```python
from build123d import *

# Parameters (mm, degrees)
RESSALTO_EXTRUS_O1_DEPTH = 17
ESBO_O2_W                = 18
ESBO_O2_H                = 13
CORTE_EXTRUS_O1_DEPTH    = 18
ESBO_O3_R                = 3
CORTE_EXTRUS_O2_DEPTH    = 2
ESBO_O4_R                = 3
CORTE_EXTRUS_O3_DEPTH    = 3


with BuildPart() as part:
    # Esboço1 → Ressalto-extrusão1 (new body)
    with BuildSketch(Plane.XY):
        Polygon((0, 0), (0, 20), (2, 20), (20, 2), (20, 0), align=None)
    extrude(amount=RESSALTO_EXTRUS_O1_DEPTH)

    # Esboço2 → Corte-extrusão1 (cut)
    with BuildSketch(Plane(origin=(0, 20, 0), x_dir=(1, 0, 0), z_dir=(0, 1, 0))):
        with Locations((11, -8.5)):
            Rectangle(ESBO_O2_W, ESBO_O2_H)
    extrude(amount=-CORTE_EXTRUS_O1_DEPTH, mode=Mode.SUBTRACT)

    # Esboço3 → Corte-extrusão2 (cut)
    with BuildSketch(Plane(origin=(2, 0, 0), x_dir=(0, 0, -1), z_dir=(1, 0, 0))):
        with Locations((-8.5, 11)):
            Circle(ESBO_O3_R)
    extrude(amount=-CORTE_EXTRUS_O2_DEPTH, mode=Mode.SUBTRACT)

    # Esboço4 → Corte-extrusão3 (cut, through all)
    with BuildSketch(Plane(origin=(0, 2, 0), x_dir=(1, 0, 0), z_dir=(0, 1, 0))):
        with Locations((11, -8.5)):
            Circle(ESBO_O4_R)
    extrude(amount=-CORTE_EXTRUS_O3_DEPTH, mode=Mode.SUBTRACT)


solid = part.part
```
Work out the finished part from the listing and answer in its coordinate system (mm). A direction names the side the tool comes from. Give positions to 0.01 mm unless a question says otherwise; leave off trailing zeros. Loops run counter-clockwise (first coordinate to the right, second up) from the corner with the lowest first, then second, coordinate; pieces in that order, holes last. Notation, with made-up numbers: (-13.75, 60) - (35.25, 60) arc R14 ccw to (35.25, 72) - close; hole circle Ø6 at (7.25, -24.75). An arc over 180 degrees is marked (long way). Use CSV: the item, a comma, the result in double quotes. Start each with the question number.
(1) Find section C-C, the plane y = 4. Determine the outline of the cut face in (x, z).
(2) Find the intervals of material crossed by L1, parallel to Z at x = 11.5, y = 6.5; L2, parallel to Z at x = 11, y = 1.5; L3, parallel to Y at x = 0.65, z = 8.5, in increasing order.
(3) Find section B-B, the plane z = 8.5. Determine the outline of the cut face in (x, y).
(4) A tool of negligible diameter and unlimited length cuts with its end or side. For faces 4 (the face through (7, 7, 2)), 5 (the face through (1.01, 9.85, 5.73)), from which of +Z, -Z, +X, -X, +Y, -Y can it reach the whole face along a straight path? Write none if from no direction.
(5) Find section D-D, the plane x = 18.25. Determine the outline of the cut face in (y, z).
(6) Find section A-A, the plane x = 11. Determine the outline of the cut face in (y, z), plus the area to 3 significant figures.
(7) Each of these flat-tipped pins is pushed along its axis until it touches: pin 1 (8 mm diameter, centred on x = 11, z = 8.5, fed in from +Y); pin 2 (4 mm diameter, centred on x = 12.5, z = 13.5, fed in from +Y); pin 3 (5 mm diameter, centred on y = 11, z = 8.5, fed in from +X); pin 4 (1 mm diameter, centred on y = 17, z = 8, fed in from +X). Where does it stop, or does it pass through?
(8) Determine the mould class of faces 1 (the face through (11, 11, 16)), 2 (the face through (8.79, 1.01, 6.47)), 3 (the face through (8, 8, 17)) for opening direction X: released by +X, released by -X, zero draft, split by the parting line, or undercut.
Results found:
1,outline,"(0, 0) - (18, 0) - (18, 2) - (2, 2) - (2, 15) - (18, 15) - (18, 17) - (0, 17) - close"
2,L1,"0 to 2, 15 to 17"
2,L2,"0 to 5.5, 11.5 to 17"
2,L3,"0 to 8, 14 to 20"
3,outline,"(0, 0) - (8, 0) - (8, 2) - (2, 2) - (2, 8) - (0, 8) - close; (0, 14) - (2, 14) - (2, 20) - (0, 20) - close; (14, 0) - (20, 0) - (20, 2) - (14, 2) - close"
4,face 4,"+X, +Y"
4,face 5,"+X, -X"
5,outline,"(0, 0) - (3.75, 0) - (3.75, 2) - (2, 2) - (2, 15) - (3.75, 15) - (3.75, 17) - (0, 17) - close"
6,outline,"(0, 0) - (11, 0) - (11, 2) - (2, 2) - (2, 5.5) - (0, 5.5) - close; (0, 11.5) - (2, 11.5) - (2, 15) - (11, 15) - (11, 17) - (0, 17) - close"
6,area,"58.0 mm^2"
7,pin 1,"y = 2"
7,pin 2,"y = 10.82"
7,pin 3,"through"
7,pin 4,"x = 2"
8,face 1,"released by +X"
8,face 2,"undercut"
8,face 3,"zero draft"
